Here's the drawing with two shaded views (mm, measured from the low corner). I have some questions. A direction names the side the tool comes from. Round coordinates to 2 decimals unless told otherwise and drop trailing zeros. Loops run counter-clockwise (first coordinate to the right, second up) from the corner with the lowest first, then second, coordinate; pieces in that order, holes last. Notation, with made-up numbers: M 31,13 L 42,13 A20 cw 42,39 Z; hole C 61.25,40.25 d2. An arc over 180 degrees is marked long. Write each question's results on one line, items separated by ' | '. Start each with the question number.
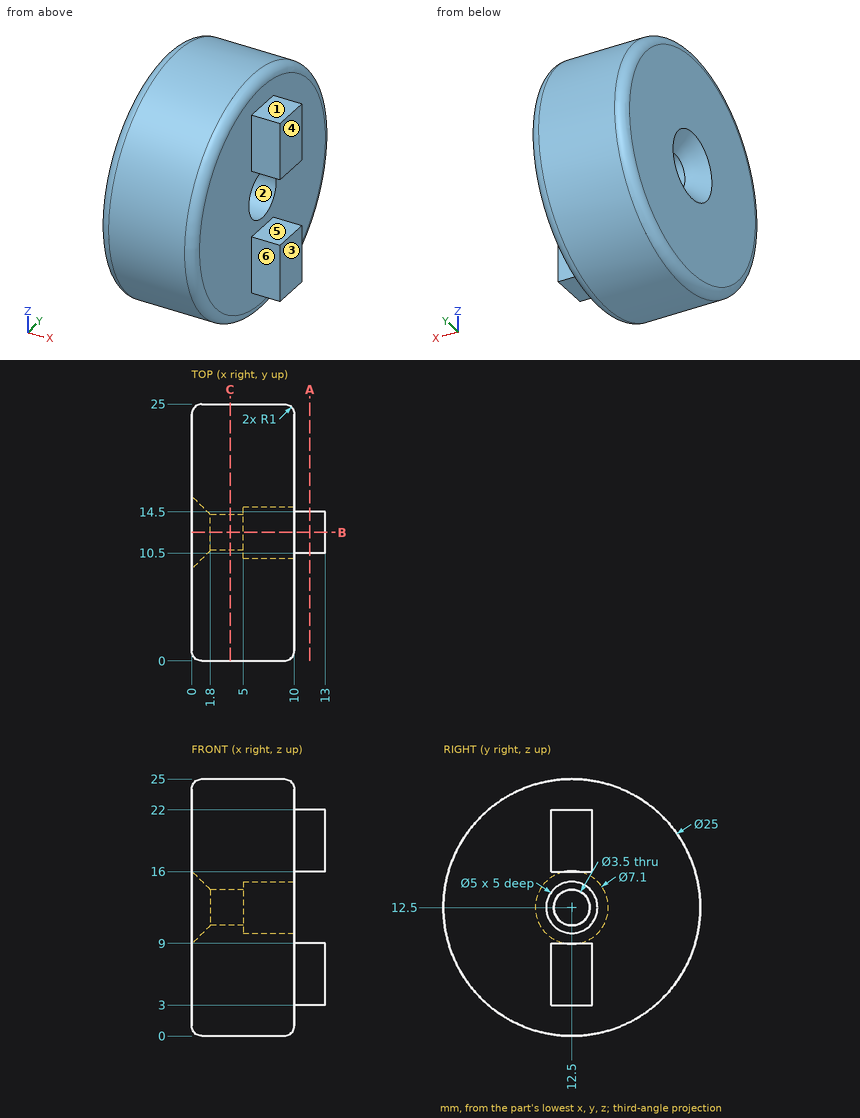
Item 1: If we section it at C-C on x = 3.75: Please give me the cut outline in (y, z), and give its area (3 significant figures).
Item 2: I need wall thicknesses on L1, parallel to Z at x = 7.75, y = 12.5; L2, parallel to Z at x = 3, y = 12.5. Which ranges of each line are inside material? Lowest first, please.
Item 3: I'm going to push flat-ended pins straight in: pin 1 (1.5 mm diameter, centred on x = 1.5, z = 4, fed in from -Y); pin 2 (1.5 mm diameter, centred on x = 1.5, y = 14, fed in from -Z); pin 3 (5 mm diameter, centred on x = 4.5, z = 6.5, fed in from +Y); pin 4 (5 mm diameter, centred on x = 8, y = 11.5, fed in from +Z). Where does each tip first touch, or does it pass through?
Item 4: If we section it at B-B on y = 12.5: Please give me the cut outline in (x, z), and give its area (3 significant figures).
Item 5: If we mould it in two halves opening along Z, with no side actions, what happens to the marked faces 1, 2 and 3? For each: released by +Z, released by -Z, zero draft, split by the parting line, or undercut.
Item 6: If we section it at A-A on x = 11.5: Please give me the cut outline in (y, z).
Item 7: Which directions (+Z, -Z, +X, -X, +Y, -Y) give clear straight access to the entire face, cutting with the end or side of a thin tool? Please do the marked faces 4, 5 and 6.
Numbers:
1) outline: C 12.5,12.5 d25; hole C 12.5,12.5 d3.5 | area: 481 mm²
2) L1: 0 to 10, 15 to 25 | L2: 0 to 10.75, 14.25 to 25
3) pin 1: y = 2.69 | pin 2: z = 0.02 | pin 3: y = 24.5 | pin 4: z = 25
4) outline: M 0,1 A1 ccw 1,0 L 9,0 A1 ccw 10,1 L 10,3 L 13,3 L 13,9 L 10,9 L 10,10 L 5,10 L 5,10.75 L 1.8,10.75 L 0,8.95 Z; M 0,16.05 L 1.8,14.25 L 5,14.25 L 5,15 L 10,15 L 10,16 L 13,16 L 13,22 L 10,22 L 10,24 A1 ccw 9,25 L 1,25 A1 ccw 0,24 Z | area: 239 mm²
5) face 1: released by +Z | face 2: undercut | face 3: zero draft
6) outline: M 10.5,3 L 14.5,3 L 14.5,9 L 10.5,9 Z; M 10.5,16 L 14.5,16 L 14.5,22 L 10.5,22 Z
7) face 4: +Z, -Z, +X, +Y, -Y | face 5: +X, +Y, -Y | face 6: +Z, -Z, +X, -Y
